Autodesk Inventor part; units mm, degrees
ref_plane "YZ Plane" through (0, 0, 0) normal (1, 0, 0) x (0, 1, 0)
ref_plane "XZ Plane" through (0, 0, 0) normal (0, 1, 0) x (-1, 0, 0)
ref_plane "XY Plane" through (0, 0, 0) normal (0, 0, 1) x (1, 0, 0)
sketch "Sketch1" plane through (0, 0, 0) normal (0, 1, 0) x (-1, 0, 0)
  circle A0 centre (0, 0) radius 12.5
  dimension "d0" = 25
extrude "Extrusion1" add sketch "Sketch1" along normal blind 19
sketch "Sketch2" plane through (0, 0, 0) normal (0, -1, 0) x (1, 0, 0)
  circle A0 centre (0, 0) radius 12.2
  dimension "d3" = 24.4
extrude "Extrusion2" add sketch "Sketch2" along normal blind 30.8
sketch "Sketch3" plane through (0, 19, 0) normal (0, 1, 0) x (1, 0, 0)
  circle A0 centre (0, 0) radius 3.5
  dimension "d6" = 7
extrude "Extrusion3" add sketch "Sketch3" along normal blind 2.5
sketch "Sketch4" plane through (0, 21.5, 0) normal (0, 1, 0) x (1, 0, 0)
  circle A0 centre (0, 0) radius 3.5
  circle A1 centre (0, 0) radius 2
  dimension "d9" = 4
extrude "Extrusion4" add sketch "Sketch4" along normal blind 10 contours A1
sketch "Sketch5" plane through (0, 19, 0) normal (0, 1, 0) x (1, 0, 0)
  circle A0 centre (0, 8.5) radius 1.65
  circle A1 centre (-8.5, 0) radius 1.65
  circle A2 centre (0, -8.5) radius 1.65
  circle A3 centre (8.5, 0) radius 1.65
  point P0 (0, 0)
  dimension "d13" = 3.3
  dimension "d16" = 360
extrude "Extrusion5" cut sketch "Sketch5" against normal blind 5
properties part number "Motor" material "Iron, Malleable"
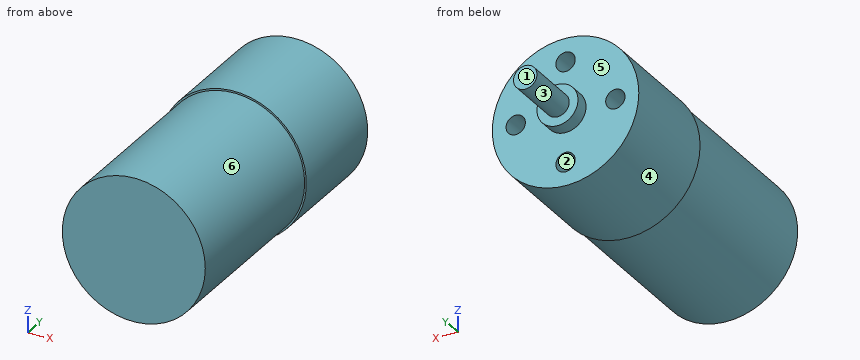
Model file for the job. Use its own axes, mm. Face numbers are marked on the shaded views. A direction names the side the tool comes from. Round coordinates to 2 decimals unless told otherwise and drop trailing zeros. Loops run counter-clockwise (first coordinate to the right, second up) from the corner with the lowest first, then second, coordinate; pieces in that order, holes last. Notation, with made-up numbers: M 36,-23 L 48,-23 A17 ccw 48,-11 Z; hole C 54,12.25 d4. An arc over 180 degrees is marked long. One line per question, with ' | ' between items.
1) Band-saw the part on B-B (y = -23). Give the cut face in (x, z), then the cut area to 3 significant figures.
Solved:
outline: C 0,0 d24.4 | area: 468 mm²
2) Flat gauge pins, fed straight in: pin 1 (4.5 mm diameter, centred on x = 0, z = 8.5, fed in from +Y); pin 2 (1.6 mm diameter, centred on x = 0, z = 8.5, fed in from +Y); pin 3 (3 mm diameter, centred on y = 19.5, z = -5, fed in from -X). Where does each tip first touch, or does it go through?
Solved:
pin 1: stops at y = 19 | pin 2: stops at y = 14 | pin 3: stops at x = -11.97
3) Band-saw the part on A-A (x = 0). Give the cut face in (y, z), then the cut area to 3 significant figures.
Solved:
outline: M -30.8,-12.2 L 0,-12.2 L 0,-12.5 L 19,-12.5 L 19,-10.15 L 14,-10.15 L 14,-6.85 L 19,-6.85 L 19,-3.5 L 21.5,-3.5 L 21.5,-2 L 31.5,-2 L 31.5,2 L 21.5,2 L 21.5,3.5 L 19,3.5 L 19,6.85 L 14,6.85 L 14,10.15 L 19,10.15 L 19,12.5 L 0,12.5 L 0,12.2 L -30.8,12.2 Z | area: 1,250 mm²
4) Mould opens along Z. For the marked faces 1, 2 and 3 say: +Z half, -Z half, draft (parallel to the pull), parting line (faces both ways), or undercut.
Solved:
face 1: draft | face 2: undercut | face 3: parting line
5) 3-axis set-ups, long thin cutter, end or side, ignore diameter. For the marked faces 4, 5 and 6: which of +Z, -Z, +X, -X, +Y, -Y reach the whole face in a straight line?
Solved:
face 4: +Y, -Y | face 5: +Y | face 6: -Y
6) Band-saw the part on C-C (z = 8.5). Give the cut face in (x, y).
Solved:
outline: M -9.17,0 L -8.75,0 L -8.75,-30.8 L 8.75,-30.8 L 8.75,0 L 9.17,0 L 9.17,19 L 1.65,19 L 1.65,14 L -1.65,14 L -1.65,19 L -9.17,19 Z
7) Band-saw the part on D-D (x = 9.5). Give the cut face in (y, z), then the cut area to 3 significant figures.
Solved:
outline: M -30.8,-7.65 L 0,-7.65 L 0,-8.12 L 19,-8.12 L 19,-1.31 L 14,-1.31 L 14,1.31 L 19,1.31 L 19,8.12 L 0,8.12 L 0,7.65 L -30.8,7.65 Z | area: 767 mm²
8) Drill centre lines: line 1 along Z through (x, y) = (0, 17.65); line 2 along Y through (x, z) = (5, -10); line 3 along Y through (x, z) = (-1, 3.25). Where is each one in solid material? Low to high.
Solved:
line 1: z = -12.5 to -10.15, -6.85 to 6.85, 10.15 to 12.5 | line 2: y = -30.8 to 19 | line 3: y = -30.8 to 21.5
